The figure shows three views and two pictorial views of one solid part (mm, origin at its lowest corner). Answer the questions. Coordinates: 2 decimals unless noted, no trailing zeros. Order: outer loops, then holes, each group sorted by start corner. A loop starts at its lowest first (then second) coordinate and runs counter-clockwise, first axis right, second up. Notation, with made-up numbers: (8.25, -11.75) - (66.25, -11.75) arc R24 cw to (66.25, 27.25) - close; hole circle Ø8 at (41.25, 49.5). An arc over 180 degrees is marked (long way). Answer as a JSON object with one key per item and string values. Group by question number.
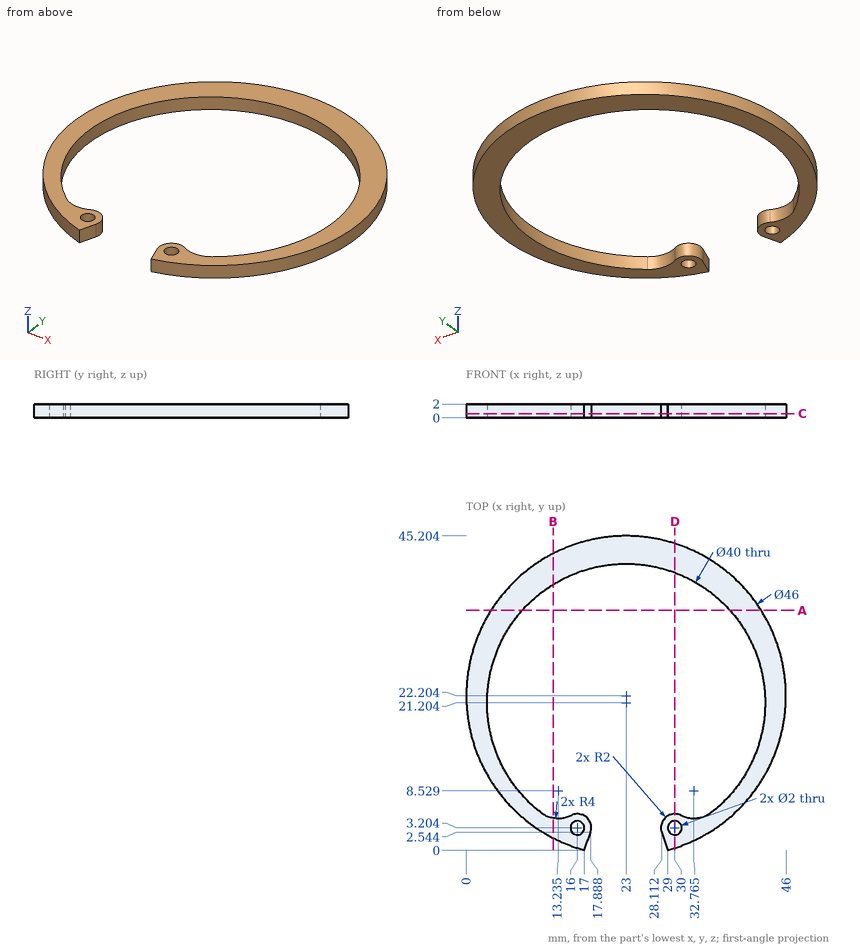
1. A cutting plane is placed at A-A on y = 34.5. Write down the section's boundary in (x, z).
2. A cutting plane is placed at B-B on x = 12.5. Write down the section's boundary in (y, z) (1 decimal).
3. A cutting plane is placed at C-C on z = 0.6. Write down the section's boundary in (x, y) (1 decimal), and give its area (3 significant figures).
4. Straight lines are drawn through the part: L1, parallel to Y at x = 30, z = 1.05 (1 decimal); L2, parallel to Y at x = 23, z = 1.6; L3, parallel to Y at x = 35, z = 0.9 (1 decimal). For each, find the intervals that lie inside material, in ascending order.
5. A cutting plane is placed at D-D on x = 30. Write down the section's boundary in (y, z) (1 decimal).
Derived:
{
 "1": {"outline": "(3.56, 0) - (8.06, 0) - (8.06, 2) - (3.56, 2) - close; (37.94, 0) - (42.44, 0) - (42.44, 2) - (37.94, 2) - close"},
 "2": {"outline": "(1.7, 0) - (4.6, 0) - (4.6, 2) - (1.7, 2) - close; (38.2, 0) - (42.7, 0) - (42.7, 2) - (38.2, 2) - close"},
 "3": {"outline": "(10.8, 5.4) arc R20 cw (long way) to (35.2, 5.4) arc R4 cw to (30.9, 5) arc R2 ccw to (28.1, 2.5) - (29, 0) arc R23 ccw (long way) to (17, 0) - (17.9, 2.5) arc R2 ccw to (15.1, 5) arc R4 cw to start; hole circle Ø2 at (16, 3.2); hole circle Ø2 at (30, 3.2)", "area": "397 mm2"},
 "4": {"L1": "y = 0.3 to 2.2, 4.2 to 5.2, 39.9 to 44.1", "L2": "y = 41.2 to 45.2", "L3": "y = 2.6 to 5.2, 37.2 to 41.8"},
 "5": {"outline": "(0.3, 0) - (2.2, 0) - (2.2, 2) - (0.3, 2) - close; (4.2, 0) - (5.2, 0) - (5.2, 2) - (4.2, 2) - close; (39.9, 0) - (44.1, 0) - (44.1, 2) - (39.9, 2) - close"}
}
